Read the model definition and answer for the solid it produces. Units are mm, in the model's axes. Face numbers are marked on the shaded views. A direction names the side the tool comes from. Round coordinates to 2 decimals unless told otherwise and drop trailing zeros. Order: outer loops, then holes, each group sorted by start corner. A loop starts at its lowest first (then second) coordinate and runs counter-clockwise, first axis right, second up. Notation, with made-up numbers: (56.5, 51) - (84.5, 51) arc R31 cw to (84.5, 81) - close; hole circle Ø1 at (-38.5, 30.5). An arc over 180 degrees is marked (long way). One line per question, with ' | ' between items. Start each with the question number.
1) Straight lines are drawn through the part: line 1 (X direction, y = -20.5, z = -7); line 2 (X direction, y = 3, z = 4); line 3 (X direction, y = 27.5, z = -2.5). For each, find the intervals that lie inside material, in ascending order. Write a range as from..to.
2) The part is cut by section A-A, the plane y = -14. Give the vertices of the cut face in (x, z).
3) For the marked faces 4 and 5, determine the directions among +Z, -Z, +X, -X, +Y, -Y from which every point of the face is accessible in a straight line to the end or side of a thin tool.
4) The part is cut by section D-D, the plane x = -4. Give the vertices of the cut face in (y, z), plus the area to 3 significant figures.
5) The part is cut by section B-B, the plane z = 0. Give the vertices of the cut face in (x, y).
6) The mould has two halves that part along X. Classify the marked faces 1, 2 and 3: pulls with the +X half, pulls with the -X half, needs draft (parallel to the pull), parting line crosses it, or undercut.
7) The part is cut by section C-C, the plane y = 10.5. Give the vertices of the cut face in (x, z), plus the area to 3 significant figures.
8) A flat-ended cylindrical pin translates along its axis: pin 1 (2 mm diameter, centred on y = 25, z = 11, fed in from +X). Find the tip coordinate at first contact, or state that the pin passes through.
from build123d import *

# Parameters (mm, degrees)
F1_DEPTH = 15.9
F2_DEPTH = 31.2
F3_R     = 10.139696962


with BuildPart() as f1:
    # F0 (on Top) → F1 (new body)
    with BuildSketch(Plane.XY):
        Polygon((-14.9499792606, 36.5612395108), (-37.1546074748, 36.5612395108), (-37.1546074748, -38.338817656), (-14.9499792606, -38.338817656), (-14.9499792606, 13.1299823828), (0, 0), (11.5315502696, 13.1299823828), (11.5315502696, -38.338817656), (32.4177630246, -38.338817656), (32.4177630246, 36.5612395108), (8.9689589565, 36.5612395108), (0, 24.0256660507), align=None)
    extrude(amount=F1_DEPTH)

    # F2 (add): a face of the model
    f2_faces = [f1.faces().sort_by_distance(p)[0] for p in [
        (-2.5598021431, 2.3799510678, 15.9),
    ]]
    extrude(f2_faces, amount=-F2_DEPTH)

    # F3
    f3_edges = [f1.edges().sort_by_distance(p)[0] for p in [
        (-26.052293, 36.56124, 15.9),
        (20.693361, 36.56124, 15.9),
        (32.417763, -0.888789, 15.9),
        (-37.154607, -0.888789, 15.9),
        (-37.154607, 36.56124, 0.3),
        (32.417763, 36.56124, 0.3),
    ]]
    fillet(f3_edges, radius=F3_R)


solid = f1.part
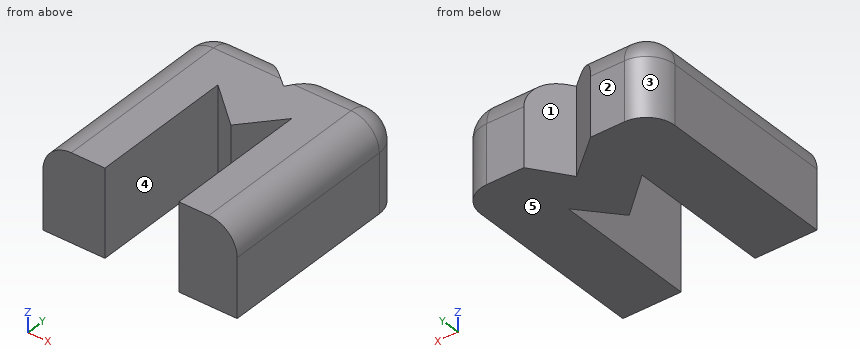
Values:
1) line 1: x = -37.15..-14.95, 11.53..32.42 | line 2: x = -37.15..-14.95, -3.42..2.63, 11.53..32.42 | line 3: x = -37.1..-4.14, 2.49..32.36
2) outline: (-37.15, -15.3) - (-14.95, -15.3) - (-14.95, 15.9) - (-27.01, 15.9) arc R10.14 ccw to (-37.15, 5.76) - close; (11.53, -15.3) - (32.42, -15.3) - (32.42, 5.76) arc R10.14 ccw to (22.28, 15.9) - (11.53, 15.9) - close
3) face 4: +Z, -Z, -Y | face 5: -Z, +X, -X, +Y, -Y
4) outline: (3.51, -15.3) - (27.38, -15.3) - (27.38, 15.85) arc R10.14 ccw to (26.42, 15.9) - (3.51, 15.9) - close | area: 745 mm^2
5) outline: (-37.15, -38.34) - (-14.95, -38.34) - (-14.95, 13.13) - (0, 0) - (11.53, 13.13) - (11.53, -38.34) - (32.42, -38.34) - (32.42, 26.42) arc R10.14 ccw to (22.28, 36.56) - (8.97, 36.56) - (0, 24.03) - (-14.95, 36.56) - (-27.01, 36.56) arc R10.14 ccw to (-37.15, 26.42) - close
6) face 1: undercut | face 2: needs draft | face 3: pulls with the -X half
7) outline: (-37.15, -15.3) - (-14.95, -15.3) - (-14.95, 15.9) - (-27.01, 15.9) arc R10.14 ccw to (-37.15, 5.76) - close; (-11.96, -15.3) - (9.22, -15.3) - (9.22, 15.9) - (-11.96, 15.9) - close; (11.53, -15.3) - (32.42, -15.3) - (32.42, 5.76) arc R10.14 ccw to (22.28, 15.9) - (11.53, 15.9) - close | area: 1,960 mm^2
8) pin 1: stops at x = 31.49
